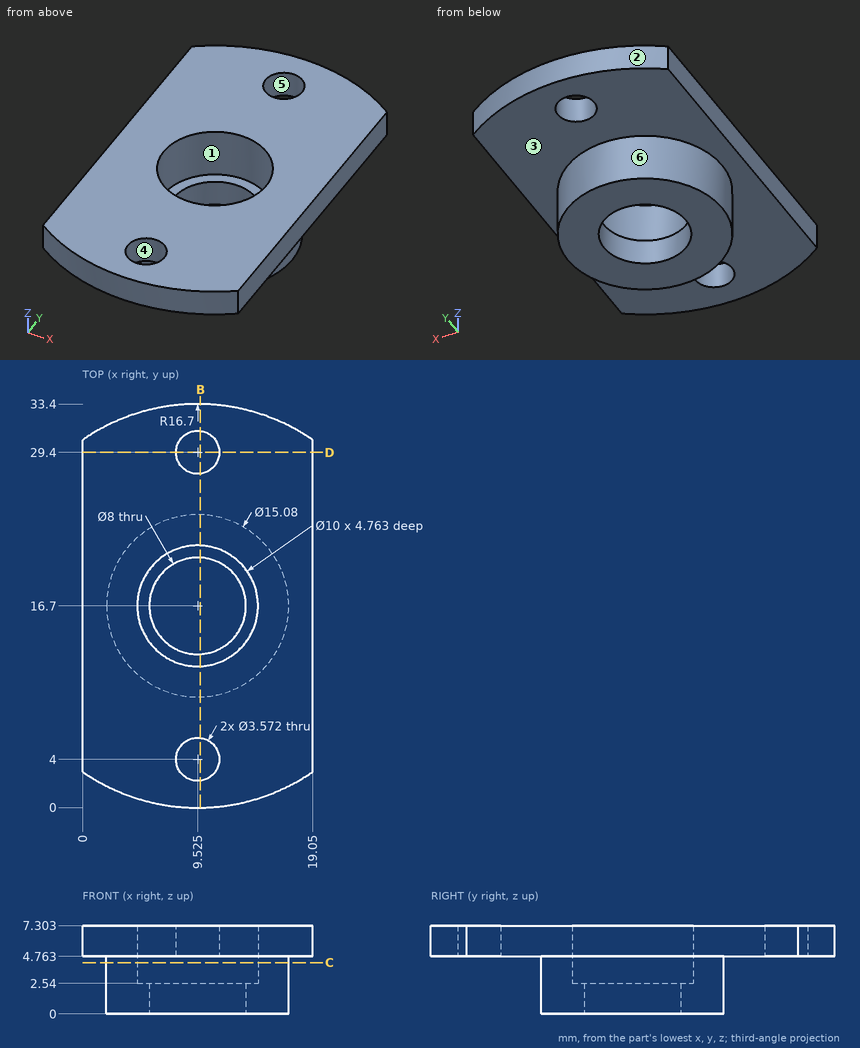
Geometry check sheet. Reference: drawing and pictorial views, mm from the part's lowest x, y, z. A direction names the side the tool comes from. Round coordinates to 2 decimals unless told otherwise and drop trailing zeros. Write each loop counter-clockwise with the first axis right and the second up, starting at its lowest first coordinate (ties: lowest second). Pieces come first, ordered by that corner, then holes.
Item 1: Section check B-B (x = 9.75). Record the boundary of the cut face in (y, z) (1 decimal).
Determined:
outline: (0, 4.8) - (2.2, 4.8) - (2.2, 7.3) - (0, 7.3) - close; (5.8, 4.8) - (9.2, 4.8) - (9.2, 0) - (12.7, 0) - (12.7, 2.5) - (11.7, 2.5) - (11.7, 7.3) - (5.8, 7.3) - close; (20.7, 0) - (24.2, 0) - (24.2, 4.8) - (27.6, 4.8) - (27.6, 7.3) - (21.7, 7.3) - (21.7, 2.5) - (20.7, 2.5) - close; (31.2, 4.8) - (33.4, 4.8) - (33.4, 7.3) - (31.2, 7.3) - close
Item 2: Material ranges on line 1 along X through (y, z) = (16.7, 1.5) (1 decimal); line 2 along Z through (x, y) = (9.5, 32); line 3 along Y through (x, z) = (8, 2) (1 decimal), recorded low to high.
Determined:
line 1: x = 2 to 5.5, 13.5 to 17.1
line 2: z = 4.76 to 7.3
line 3: y = 9.3 to 13, 20.4 to 24.1
Item 3: Access from +Z, -Z, +X, -X, +Y, -Y to the whole of each face (thin tool, end or side, straight path). Record for the marked faces 1 and 2.
Determined:
face 1: +Z
face 2: +Z, -Z, +Y
Item 4: Go/stop test with a flat-tipped pin: pin 1 Ø5.5 at (x, y) = (9.525, 4) entering from -Z. Record where the tip stops, or that it passes through.
Determined:
pin 1: stops at z = 4.76
Item 5: Mould release check, pull along X, two halves, no side actions. Record for the marked faces 3, 4, 5 and 6: +X half, -X half, draft (parallel to the pull), parting line (faces both ways), or undercut.
Determined:
face 3: draft
face 4: undercut
face 5: undercut
face 6: parting line
Item 6: Section check C-C (z = 4.25). Record the boundary of the cut face in (x, y) (1 decimal).
Determined:
outline: circle Ø15.1 at (9.5, 16.7); hole circle Ø10 at (9.5, 16.7)
Item 7: Section check D-D (y = 29.4). Record the boundary of the cut face in (x, z).
Determined:
outline: (0, 4.76) - (7.74, 4.76) - (7.74, 7.3) - (0, 7.3) - close; (11.31, 4.76) - (19.05, 4.76) - (19.05, 7.3) - (11.31, 7.3) - close
